Design review of the part built by this model. Coordinates are the model's own, in mm. Face numbers are marked on the shaded views. A direction names the side the tool comes from. Coordinates: 2 decimals unless noted, no trailing zeros. Order: outer loops, then holes, each group sorted by start corner. A loop starts at its lowest first (then second) coordinate and runs counter-clockwise, first axis right, second up. Notation, with made-up numbers: M -28,87 L -10,87 A27 ccw -10,125 Z; hole C -9,60.5 d8. An arc over 180 degrees is marked long. Answer as a JSON object with one key per item and string values.
from build123d import *
from build123d.topology import SkipClean

# Parameters (mm, degrees)
CROQUIS1_R               = 1.5875
SALIENTE_EXTRUIR1_DEPTH  = 3.175
CORTAR_EXTRUIR1_DEPTH    = 3.175
CORTAR_EXTRUIR3_DEPTH    = 10
CROQUIS4_R               = 10
CORTAR_EXTRUIR4_DEPTH    = 10
REDONDEO1_R              = 2
BOSS_EXTRUDE1_DEPTH      = 26.82
BOSS_EXTRUDE2_DEPTH      = 2
BOSS_EXTRUDE5_REACH      = 56.057
BOSS_EXTRUDE5_END_RADIUS = 10
SKETCH6_W                = 4
SKETCH6_H                = 4
SKETCH7_W                = 0.75
SKETCH7_H                = 0.75
SKETCH7_W_2              = 0.804911675
BOSS_EXTRUDE6_DEPTH      = 3
LPATTERN1_COUNT          = 4
LPATTERN1_PITCH          = 7


with BuildPart() as part:
    # Croquis1 → Saliente-Extruir1 (new body)
    with BuildSketch(Plane(origin=(0, 0, 0), x_dir=(1, 0, 0), z_dir=(0, 1, 0))):
        with BuildLine():
            Line((-12.5, 0), (-12.5, -40))
            Line((-12.5, -40), (-2.975, -40))
            Line((-2.975, -40), (-2.975, -20))
            ThreePointArc((-2.975, -20), (-0.046067812, -12.928932188), (7.025, -10))
            Line((7.025, -10), (12.5, -10))
            Line((12.5, -10), (12.5, 40))
            Line((12.5, 40), (2.5, 40))
            Line((2.5, 40), (-12.5, 0))
        make_face()
        with Locations(Location((-7.7375, -5, 0), (0, 0, 270))):
            Circle(CROQUIS1_R, mode=Mode.SUBTRACT)
        with Locations(Location((-7.7375, -35, 0), (0, 0, 270))):
            Circle(CROQUIS1_R, mode=Mode.SUBTRACT)
    extrude(amount=SALIENTE_EXTRUIR1_DEPTH)

    # Croquis2 → Cortar-Extruir1 (cut)
    with BuildSketch(Plane(origin=(0, 3.175, 0), x_dir=(1, 0, 0), z_dir=(0, 1, 0))):
        Polygon((12.5, -10), (6.1, 40), (12.5, 40), align=None)
    extrude(amount=-CORTAR_EXTRUIR1_DEPTH, mode=Mode.SUBTRACT)

    # Croquis3 → Cortar-Extruir3 (cut)
    with BuildSketch(Plane(origin=(0, 3.175, 0), x_dir=(1, 0, 0), z_dir=(0, 1, 0))):
        with BuildLine():
            ThreePointArc((-5.975, -30.575635639), (-7.7375, -30.2375), (-9.5, -30.575635639))
            Line((-9.5, -30.575635639), (-9.5, -9.427055314))
            ThreePointArc((-9.5, -9.427055314), (-7.7375, -9.765), (-5.975, -9.427055314))
            Line((-5.975, -9.427055314), (-5.975, -14.803847577))
            Line((-5.975, -14.803847577), (-5.975, -30.575635639))
        make_face()
        with BuildLine():
            ThreePointArc((-12.5, -35), (-7.7375, -39.7625), (-2.975, -35))
            Line((-2.975, -35), (-2.975, -40))
            Line((-2.975, -40), (-12.5, -40))
            Line((-12.5, -40), (-12.5, -35))
        make_face()
    extrude(amount=-CORTAR_EXTRUIR3_DEPTH, mode=Mode.SUBTRACT)

    # Croquis4 → Cortar-Extruir4 (cut)
    with BuildSketch(Plane(origin=(0, 3.175, 0), x_dir=(1, 0, 0), z_dir=(0, 1, 0))):
        with Locations((9.274103387, 15.202317292)):
            Circle(CROQUIS4_R)
        Polygon((7.025, -10), (11.878723404, -5.146276596), (12.5, -10), align=None)
    extrude(amount=-CORTAR_EXTRUIR4_DEPTH, mode=Mode.SUBTRACT)

    # Redondeo1
    redondeo1_edges = [part.edges().sort_by_distance(p)[0] for p in [
        (8.004462032, 1.5875, -25.121390375),
        (10.543744741, 1.5875, -5.283244209),
    ]]
    fillet(redondeo1_edges, radius=REDONDEO1_R)

    # Sketch1 → Boss-Extrude1 (add)
    with SkipClean():  # the faces are left unmerged after this step: merging them gives an invalid solid
        with BuildSketch(Plane(origin=(0, 3.175, 0), x_dir=(1, 0, 0), z_dir=(0, 1, 0))):
            with BuildLine():
                Line((7.771843477, 26.938722839), (5.78802886, 26.684794568))
                ThreePointArc((5.78802886, 26.684794568), (-2.628784313, 13.678747666), (8.79254868, 3.211983474))
                Line((8.79254868, 3.211983474), (10.776363297, 3.465911745))
                ThreePointArc((10.776363297, 3.465911745), (10.143802127, 4.686471223), (8.872807798, 5.210372444))
                ThreePointArc((8.872807798, 5.210372444), (-0.644969697, 13.932675937), (6.369041281, 24.771048355))
                ThreePointArc((6.369041281, 24.771048355), (7.467102295, 25.59818866), (7.771843477, 26.938722839))
            make_face()
        extrude(amount=BOSS_EXTRUDE1_DEPTH)

    # Sketch2 → Boss-Extrude2 (add)
    with SkipClean():  # the faces are left unmerged after this step: merging them gives an invalid solid
        with BuildSketch(Plane(origin=(0, 29.995, 0), x_dir=(1, 0, 0), z_dir=(0, 1, 0))):
            with BuildLine():
                Line((10.776363297, 3.465911745), (7.771843477, 26.938722839))
                Line((7.771843477, 26.938722839), (5.78802886, 26.684794568))
                ThreePointArc((5.78802886, 26.684794568), (-2.628784313, 13.678747666), (8.79254868, 3.211983474))
                Line((8.79254868, 3.211983474), (10.776363297, 3.465911745))
            make_face()
        extrude(amount=BOSS_EXTRUDE2_DEPTH)

    # Boss-Extrude5: up to this cylinder (the profile starts inside it)
    with SkipClean():  # the faces are left unmerged after this step: merging them gives an invalid solid
        boss_extrude5_end = Plane(origin=(9.274103387, 26.995, -15.202317292), z_dir=(0, 1, 0)) * Cylinder(BOSS_EXTRUDE5_END_RADIUS, 133.114, mode=Mode.PRIVATE)
        # Sketch6 → Boss-Extrude5 (add, up to the surface)
        with BuildSketch(Plane(origin=(4.095783657, 0, -0.524260308), x_dir=(-0.12696413546540503, 0, -0.9919073083234755), z_dir=(0.9919073083234755, 0, -0.12696413546540503)), mode=Mode.PRIVATE) as boss_extrude5_sk1:
            with Locations((13.901811107, 26.995)):
                Rectangle(SKETCH6_W, SKETCH6_H)
        boss_extrude5_tool1 = extrude(boss_extrude5_sk1.sketch, amount=-BOSS_EXTRUDE5_REACH, mode=Mode.PRIVATE) & boss_extrude5_end
        boss_extrude5 = boss_extrude5_tool1.solids().sort_by_distance((2.330752, 26.995, -14.313568))[0]
        add(boss_extrude5)

    # Sketch7 → Boss-Extrude6 (add)
    with SkipClean():  # the faces are left unmerged after this step: merging them gives an invalid solid
        with BuildSketch(Plane(origin=(4.095783657, 0, -0.524260308), x_dir=(-0.12696413546540503, 0, -0.9919073083234755), z_dir=(0.9919073083234755, 0, -0.12696413546540503))):
            with Locations((15.329266944, 26.995)):
                Rectangle(SKETCH7_W, SKETCH7_H)
            with Locations((13.901811107, 26.995)):
                Rectangle(SKETCH7_W_2, SKETCH7_H)
            with Locations((12.474355269, 26.995)):
                Rectangle(SKETCH7_W, SKETCH7_H)
        boss_extrude6 = extrude(amount=BOSS_EXTRUDE6_DEPTH)

    # LPattern1: Boss-Extrude5, Boss-Extrude6 ×4
    with SkipClean():  # the faces are left unmerged after this step: merging them gives an invalid solid
        with Locations(*[(0, -i * LPATTERN1_PITCH, 0) for i in range(1, LPATTERN1_COUNT)]):
            add(boss_extrude5)
            add(boss_extrude6)


solid = part.part
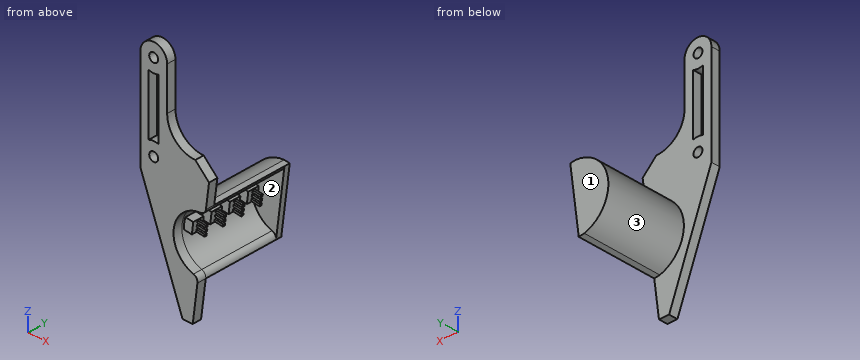
1) To check wall thickness, follow L1, parallel to X at y = 2, z = 5 (3 decimals); L2, parallel to X at y = 0.85, z = 35 (3 decimals); L3, parallel to Y at x = 7.25, z = -0.5 (3 decimals). State the ranges of each line that lie inside material, in increasing order.
Taken from the geometry:
{"L1": "x = -12.5 to -9.325, -6.15 to 11.86", "L2": "x = -12.5 to -9.325, -6.15 to -2.975", "L3": "y = 0 to 3.175"}
2) Tool access review of the marked faces 1, 2 and 3: name each direction out of +Z, -Z, +X, -X, +Y, -Y from which nothing blocks a thin tool from reaching the whole face with its end or side.
Taken from the geometry:
{"face 1": "+Z, -Z, +X, -X, +Y", "face 2": "+X", "face 3": "-X, +Y"}
3) Add section B-B (x = -4.5). State the section outline as (y, z) points (3 decimals), and give its area (3 significant figures).
Taken from the geometry:
{"outline": "M 0,-21.333 L 3.175,-21.333 L 3.175,38.493 L 0,38.493 Z", "area": "190 mm2"}
4) Add section A-A (z = -24). State the section outline as (x, y) points (3 decimals).
Taken from the geometry:
{"outline": "M -3.5,0 L 4.52,0 L 4.52,29.995 L 8.148,29.995 L 8.148,31.995 L 1.113,31.995 L 1.113,3.175 L -3.5,3.175 Z"}
5) Insertion check: pin 1 Ø1.7 at (x, z) = (1.5, -15) entering from -Y (3 decimals); pin 2 Ø6 at (x, y) = (7, 16.5) entering from +Z; pin 3 Ø0.6 at (x, z) = (4.5, -14.5) entering from -Y. Each pin has a flat end and moves straight along its axis. Give the tip position at first contact, or say it passes through.
Taken from the geometry:
{"pin 1": "stops at y = 3.995", "pin 2": "stops at z = -3.21", "pin 3": "stops at y = 5.62"}
